Design review of the part built by this model. Coordinates are the model's own, in mm. Face numbers are marked on the shaded views. A direction names the side the tool comes from. Coordinates: 2 decimals unless noted, no trailing zeros. Order: outer loops, then holes, each group sorted by start corner. A loop starts at its lowest first (then second) coordinate and runs counter-clockwise, first axis right, second up. Notation, with made-up numbers: M 0,13 L 41,13 A14 cw 41,23 Z; hole C -7,19.25 d8. An arc over 180 degrees is marked long. Answer in a Markdown table with one row per item.
from build123d import *

# Parameters (mm, degrees)
SKETCH1_R            = 3.25
BOSS_EXTRUDE1_DEPTH  = 3
EDGE_FLANGE1_DEPTH   = 32
SKETCH12_W           = 12
SKETCH12_H           = 15
BOSS_EXTRUDE2_DEPTH  = 3
EDGE_FLANGE3_DEPTH   = 12
CUT_EXTRUDE1_DEPTH   = 131.469345059
FILLET1_R            = 5
M5_CLEARANCE_HOLE1_D = 5.5


# Sheet-metal steps are written as plain solids
with BuildPart() as part:
    # Sketch1 → Boss-Extrude1 (new body)
    with BuildSketch(Plane(origin=(0, 0, 0), x_dir=(1, 0, 0), z_dir=(0, 1, 0))):
        with BuildLine():
            Line((-7.5, 0), (-7.5, 120))
            Line((-7.5, 120), (7.6, 120))
            Line((7.6, 120), (7.6, 88))
            Line((7.6, 88), (7.5, 88))
            Line((7.5, 88), (7.5, 0))
            ThreePointArc((7.5, 0), (0, -7.5), (-7.5, 0))
        make_face()
        with Locations(Location((0, 0, 0), (0, 0, 270))):
            Circle(SKETCH1_R, mode=Mode.SUBTRACT)
    extrude(amount=BOSS_EXTRUDE1_DEPTH)

    # Edge-Flange1 section (across the edge) → Edge-Flange1 (add)
    with BuildSketch(Plane(origin=(11.1, 3, -88), x_dir=(-1, 0, 0), z_dir=(0, 0, -1))):
        with BuildLine():
            Line((-3, 3.5), (-3, 17))
            Line((-3, 17), (0, 17))
            Line((0, 17), (0, 3.5))
            ThreePointArc((0, 3.5), (1.025126266, 1.025126266), (3.5, 0))
            Line((3.5, 0), (3.5, -3))
            ThreePointArc((3.5, -3), (-1.096194078, -1.096194078), (-3, 3.5))
        make_face()
    extrude(amount=EDGE_FLANGE1_DEPTH)

    # Sketch12 → Boss-Extrude2 (add)
    with BuildSketch(Plane.ZY.offset(-11.1)):
        with Locations((-94, 27.5)):
            Rectangle(SKETCH12_W, SKETCH12_H)
    extrude(amount=-BOSS_EXTRUDE2_DEPTH)

    # Edge-Flange3 section (across the edge) → Edge-Flange3 (add)
    with BuildSketch(Plane(origin=(14.1, 38.5, -100), x_dir=(0, -1, 0), z_dir=(0, 0, 1))):
        with BuildLine():
            Line((-3, 3.5), (-3, 27))
            Line((-3, 27), (0, 27))
            Line((0, 27), (0, 3.5))
            ThreePointArc((0, 3.5), (1.025126266, 1.025126266), (3.5, 0))
            Line((3.5, 0), (3.5, -3))
            ThreePointArc((3.5, -3), (-1.096194078, -1.096194078), (-3, 3.5))
        make_face()
    extrude(amount=EDGE_FLANGE3_DEPTH)

    # Sketch16 → Cut-Extrude1 (cut, through all)
    with BuildSketch(Plane.ZY.offset(-11.1)):
        with BuildLine():
            Line((-112, 15.7), (-96, 15.7))
            ThreePointArc((-96, 15.7), (-93.3, 13), (-96, 10.3))
            Line((-96, 10.3), (-112, 10.3))
            ThreePointArc((-112, 10.3), (-114.7, 13), (-112, 15.7))
        make_face()
    extrude(amount=-CUT_EXTRUDE1_DEPTH, mode=Mode.SUBTRACT)

    # Fillet1
    fillet1_edges = [part.edges().sort_by_distance(p)[0] for p in [
        (12.6, 20, -120),
        (12.6, 20, -100),
    ]]
    fillet(fillet1_edges, radius=FILLET1_R)

    # M5 Clearance Hole1 (through all)
    with Locations(Plane(origin=(0, 41.5, 0), x_dir=(1, 0, 0), z_dir=(0, 1, 0))):
        with Locations((34.1, 94)):
            Hole(M5_CLEARANCE_HOLE1_D / 2)


solid = part.part
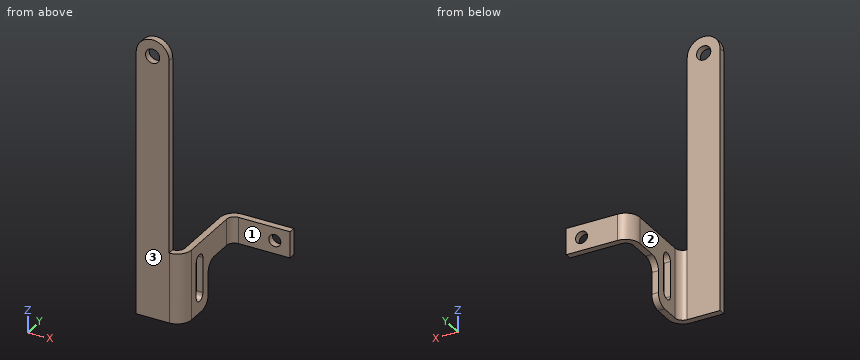
(1) For line 1 along Z through (x, y) = (34.1, 39.1); line 2 along Y through (x, z) = (5.5, -110); line 3 along Y through (x, z) = (31.5, -99), list the stretches that pass through material, from the lowest coordinate up. Write a range as from..to.
Return value:
| item | result |
|---|---|
| line 1 | z = -100..-96.75, -91.25..-88 |
| line 2 | y = 0..3 |
| line 3 | y = 38.5..41.5 |
(2) Add section A-A, the plane x = 34.1. Give the boundary of the cut face in (y, z).
Return value:
| item | result |
|---|---|
| outline | M 38.5,-100 L 41.5,-100 L 41.5,-96.75 L 38.5,-96.75 Z; M 38.5,-91.25 L 41.5,-91.25 L 41.5,-88 L 38.5,-88 Z |
(3) For the marked faces 1, 2 and 3, list the 3-axis set-ups (+Z, -Z, +X, -X, +Y, -Y) from which the entire face can be reached by the end or side of a thin tool; tool diameter is ignored.
Return value:
| item | result |
|---|---|
| face 1 | +Z, -Z, +X, -Y |
| face 2 | +Z, -Z, -X, +Y |
| face 3 | +Z, -Z, +X, -X, -Y |
(4) Insertion check: pin 1 Ø1.5 at (x, z) = (13, -105.5) entering from -Y; pin 2 Ø3.5 at (x, z) = (26, -95) entering from -Y; pin 3 Ø1.5 at (y, z) = (16.5, -95.5) entering from -X; pin 4 Ø6 at (x, z) = (0, 0) entering from +Y. Each pin has a flat end and moves straight along its axis. Give the tip position at first contact, or say it passes through.
Return value:
| item | result |
|---|---|
| pin 1 | stops at y = 1.96 |
| pin 2 | stops at y = 38.5 |
| pin 3 | stops at x = 11.1 |
| pin 4 | passes through |
(5) Add section D-D, the plane z = -31. Give the boundary of the cut face in (x, y).
Return value:
| item | result |
|---|---|
| outline | M -7.5,0 L 7.5,0 L 7.5,3 L -7.5,3 Z |
(6) Add section B-B, the plane y = 13. Give the boundary of the cut face in (x, z), and give its area (3 significant figures).
Return value:
| item | result |
|---|---|
| outline | M 11.1,-120 L 14.1,-120 L 14.1,-114.7 L 11.1,-114.7 Z; M 11.1,-93.3 L 14.1,-93.3 L 14.1,-88 L 11.1,-88 Z |
| area | 31.8 mm2 |
(7) Add section C-C, the plane x = 27. Give the boundary of the cut face in (y, z).
Return value:
| item | result |
|---|---|
| outline | M 38.5,-100 L 41.5,-100 L 41.5,-88 L 38.5,-88 Z |
